Part model, mm, in its own coordinate system. A direction names the side the tool comes from. Give positions to 0.01 mm unless a question says otherwise; leave off trailing zeros. Loops run counter-clockwise (first coordinate to the right, second up) from the corner with the lowest first, then second, coordinate; pieces in that order, holes last. Notation, with made-up numbers: (60, -3.5) -> (110, -3.5) arc R14 ccw to (110, 9.5) -> close; hole circle Ø10 at (29, 85.25). An arc over 180 degrees is marked (long way). Write item = value, one per line.
Autodesk Inventor part; units mm, degrees
ref_plane "Work Plane1" through (0, 0, 29) normal (0, 0, 1) x (1, 0, 0)
ref_plane "YZ Plane" through (0, 0, 0) normal (1, 0, 0) x (0, 1, 0)
ref_plane "XZ Plane" through (0, 0, 0) normal (0, 1, 0) x (-1, 0, 0)
sketch "Sketch1" plane through (0, 0, 0) normal (0, 0, 1) x (1, 0, 0)
  circle A0 centre (0, 0) radius 1
  dimension "d0" = 2
extrude "Extrusion1" add sketch "Sketch1" along normal blind 40 and the other way blind 3
ref_plane "Work Plane1" through (0, 0, 29) normal (0, 0, 1) x (1, 0, 0)
sketch "Sketch2" plane through (0, 0, 29) normal (0, 0, 1) x (1, 0, 0)
  circle A0 centre (0, 0) radius 1
  line L0 (-0.24, 1) -> (-0.24, 5)
  line L1 (-0.24, 5) -> (0.24, 5)
  line L2 (0.24, 5) -> (0.24, 1)
  circle A1 centre (0, 0) radius 1
  line L3 (-0.24, 1) -> (-0.24, 0.957)
  line L4 (-0.24, 0.957) -> (0.24, 0.957)
  line L5 (0.24, 0.957) -> (0.24, 1)
  dimension "d5" = 4
  dimension "d6" = 0.48
  dimension "d7" = 4
  dimension "d9" = 0.24
  dimension "d10" = 5
  dimension "d11" = 5
extrude "Extrusion2" add sketch "Sketch2" against normal blind 26 contours L5 L4 L3 A0 | A0 L3 L0 L1 L2 L5 picked at (0.0269, 0.9702)
fillet "Fillet1" radius 0.21 2 edges at (0.24, 5, 16) (-0.24, 5, 16)
pattern_circular "Circular Pattern3" count 4 over 360 about axis through (0, 0, -10) along (0, 0, 1)
chamfer "Chamfer1" distance 0.21 angle 45 2 edges at (-1, 0, 40) (-1, 0, -3)
properties part number "fan"
1) Drop flat-ended pins along their axis: P1, Ø3, axis at y = -3.5, z = 8.5, coming from the -X side; P2, Ø1.9, axis at x = -3.5, z = 10, coming from the +Y side; P3, Ø1.9, axis at y = 2, z = 14, coming from the +X side. Give the stop position or say it passes through.
Resolved:
P1 = -0.24
P2 = 0.24
P3 = 0.24
2) Which spindle directions (+Z, -Z, +X, -X, +Y, -Y) get a long thin tool onto all of the face, cutting with end or side? Do faces 1 (the face through (-3, 0.24, 16)), 2 (the face through (-3, -0.24, 16)), 3 (the face through (3, 0.24, 16)). Say none if no direction does.
Resolved:
face_1 = +Z, -Z, -X, +Y
face_2 = +Z, -Z, -X, -Y
face_3 = +Z, -Z, +X, +Y
3) Slice it at B-B, the plane x = -1.75. List the corners of the cut face in (y, z), and give its area (3 significant figures).
Resolved:
outline = (-0.24, 3) -> (0.24, 3) -> (0.24, 29) -> (-0.24, 29) -> close
area = 12.5 mm²
4) Drill centre lines: line 1 along X through (y, z) = (1.75, 7.5); line 2 along Y through (x, z) = (-0.25, 1.5). Where is each one in solid material? Low to high. Write a range as [from, to].
Resolved:
line_1 = [-0.24, 0.24]
line_2 = [-0.97, 0.97]
5) Slice it at A-A, the plane z = 8. List the corners of the cut face in (x, y), and give its area (3 significant figures).
Resolved:
outline = (-5, -0.03) arc R0.21 ccw to (-4.79, -0.24) -> (-0.97, -0.24) arc R1 ccw to (-0.24, -0.97) -> (-0.24, -4.79) arc R0.21 ccw to (-0.03, -5) -> (0.03, -5) arc R0.21 ccw to (0.24, -4.79) -> (0.24, -0.97) arc R1 ccw to (0.97, -0.24) -> (4.79, -0.24) arc R0.21 ccw to (5, -0.03) -> (5, 0.03) arc R0.21 ccw to (4.79, 0.24) -> (0.97, 0.24) arc R1 ccw to (0.24, 0.97) -> (0.24, 4.79) arc R0.21 ccw to (0.03, 5) -> (-0.03, 5) arc R0.21 ccw to (-0.24, 4.79) -> (-0.24, 0.97) arc R1 ccw to (-0.97, 0.24) -> (-4.79, 0.24) arc R0.21 ccw to (-5, 0.03) -> close
area = 10.8 mm²
